Design review of the part built by this model. Coordinates are the model's own, in mm. Face numbers are marked on the shaded views. Round coordinates to 2 decimals unless told otherwise and drop trailing zeros. Write each loop counter-clockwise with the first axis right and the second up, starting at its lowest first coordinate (ties: lowest second). Pieces come first, ordered by that corner, then holes. Notation, with made-up numbers: M 25,-11.75 L 67,-11.75 A36 ccw 67,23.25 Z; hole C 85,-34 d8. An arc over 180 degrees is marked long. One line per question, with ' | ' between items. Start each with the question number.
Item 1: Add section B-B, the plane z = 0. State the section outline as (x, y) points, and give its area (3 significant figures).
Item 2: Add section C-C, the plane y = 16.5. State the section outline as (x, z) points.
Item 3: For L1, parallel to X at y = 5, z = 9; L2, parallel to Z at x = 10, y = 3; L3, parallel to Z at x = -9.5, y = 6, list the stretches that pass through material, from the lowest coordinate up.
Item 4: Draft analysis for pull direction X (two halves, no side actions). For the marked faces 1, 2 and 3, state which applies: released by +X, released by -X, zero draft, split by the parting line, or undercut.
Item 5: Insertion check: pin 1 Ø2 at (y, z) = (17, 16) entering from +X; pin 2 Ø6 at (y, z) = (10.5, -12.5) entering from -X; pin 3 Ø4 at (x, z) = (8.5, -12.5) entering from +Y. Each pin has a flat end and moves straight along its axis. Give the tip position at first contact, or say it passes through.
Item 6: Add section A-A, the plane y = 23.5. State the section outline as (x, z) points, and give its area (3 significant figures).
```python
from build123d import *

# Parameters (mm, degrees)
SKETCH2_R           = 22
BOSS_EXTRUDE3_DEPTH = 30
SKETCH1_R           = 4.5
CUT_EXTRUDE2_DEPTH  = 25
FILLET1_R           = 7.5
BOSS_EXTRUDE4_DEPTH = 1


with BuildPart() as part:
    # Sketch2 → Boss-Extrude3 (new body)
    with BuildSketch(Plane(origin=(0, 30, 0), x_dir=(1, 0, 0), z_dir=(0, 1, 0))):
        with Locations(Location((0, 0, 0), (0, 0, 270))):
            Circle(SKETCH2_R)
    extrude(amount=-BOSS_EXTRUDE3_DEPTH)

    # Sketch1 → Cut-Extrude2 (cut)
    with BuildSketch(Plane(origin=(0, 0, 0), x_dir=(1, 0, 0), z_dir=(0, 1, 0))):
        with Locations(Location((0, 13, 0), (0, 0, 270))):
            Circle(SKETCH1_R)
        with Locations(Location((-11.258330249, 6.5, 0), (0, 0, 270))):
            Circle(SKETCH1_R)
        with Locations(Location((-11.258330249, -6.5, 0), (0, 0, 270))):
            Circle(SKETCH1_R)
        with Locations(Location((11.258330249, 6.5, 0), (0, 0, 270))):
            Circle(SKETCH1_R)
        with Locations(Location((11.258330249, -6.5, 0), (0, 0, 270))):
            Circle(SKETCH1_R)
        with Locations(Location((0, -13, 0), (0, 0, 270))):
            Circle(SKETCH1_R)
    extrude(amount=CUT_EXTRUDE2_DEPTH, mode=Mode.SUBTRACT)

    # Fillet1
    fillet1_edges = [part.edges().sort_by_distance(p)[0] for p in [
        (0, 30, -22),
    ]]
    fillet(fillet1_edges, radius=FILLET1_R)

    # Sketch3 → Boss-Extrude4 (add)
    with BuildSketch(Plane(origin=(0, 30, 0), x_dir=(1, 0, 0), z_dir=(0, 1, 0))):
        with BuildLine():
            Line((-5.047435897, 6.7), (-3.907692308, 6.7))
            Line((-3.907692308, 6.7), (-3.907692308, -1.876061699))
            add(Edge.make_bspline(
                [(-3.907692308, -1.876061699), (-3.908831384, -2.034649033), (-3.911018549, -2.339156067), (-3.923045124, -2.777755632), (-3.945300887, -3.17824355), (-3.977722218, -3.541530486), (-4.020975634, -3.86647833), (-4.070473079, -4.155597886), (-4.130390949, -4.406476162), (-4.220620698, -4.688181596), (-4.368571883, -4.997131973), (-4.591246564, -5.330797805), (-4.867862712, -5.622656181), (-5.188269318, -5.876121783), (-5.555266748, -6.078078021), (-5.961297429, -6.22305824), (-6.403861903, -6.311489634), (-6.710836188, -6.320829233), (-6.868990385, -6.325641026)],
                knots=[0, 0, 0, 0, 1.237770943, 2.376671248, 3.424123796, 4.367912054, 5.222547132, 5.982086412, 6.656319012, 7.234008312, 8.288027371, 9.317870876, 10.352700517, 11.413286737, 12.494591526, 13.606319346, 14.766767577, 16, 16, 16, 16], degree=3))
            add(Edge.make_bspline(
                [(-6.868990385, -6.325641026), (-6.992210713, -6.321719958), (-7.240138175, -6.313830511), (-7.609130176, -6.249526009), (-7.977074488, -6.150407795), (-8.345924031, -6.00525552), (-8.722966135, -5.80784092), (-9.113307336, -5.549541728), (-9.521968629, -5.230838761), (-9.791147982, -4.987587513), (-9.932051282, -4.86025641)],
                knots=[0, 0, 0, 0, 0.848567217, 1.707373443, 2.573483905, 3.470863513, 4.432650262, 5.500696352, 6.691726801, 8, 8, 8, 8], degree=3))
            Line((-9.932051282, -4.86025641), (-9.260416667, -3.883333333))
            add(Edge.make_bspline(
                [(-9.260416667, -3.883333333), (-9.105466946, -3.990185314), (-8.812901668, -4.191935786), (-8.38289984, -4.451475164), (-8.00191017, -4.673997908), (-7.75268919, -4.787399035), (-7.637299679, -4.839903846)],
                knots=[0, 0, 0, 0, 1.196737151, 2.259595785, 3.194191475, 4, 4, 4, 4], degree=3))
            add(Edge.make_bspline(
                [(-7.637299679, -4.839903846), (-7.567325178, -4.867333877), (-7.430089597, -4.921130276), (-7.220267165, -4.98116825), (-7.011642317, -5.01397928), (-6.873329542, -5.020080117), (-6.805388622, -5.023076923)],
                knots=[0, 0, 0, 0, 1.051806502, 2.062826769, 3.048436908, 4, 4, 4, 4], degree=3))
            add(Edge.make_bspline(
                [(-6.805388622, -5.023076923), (-6.717639647, -5.019365856), (-6.544192277, -5.012030446), (-6.292137213, -4.947263075), (-6.050989499, -4.848404813), (-5.829393884, -4.703656404), (-5.625158337, -4.531548106), (-5.456637227, -4.323427732), (-5.31614894, -4.092774019), (-5.231604338, -3.8744376), (-5.177739023, -3.675313828), (-5.143551977, -3.492313592), (-5.113657409, -3.278367655), (-5.087598635, -3.033220643), (-5.072342413, -2.756381753), (-5.055225452, -2.448663863), (-5.049037791, -2.109291153), (-5.047986155, -1.872668556), (-5.047435897, -1.748858173)],
                knots=[0, 0, 0, 0, 0.997221856, 1.971139923, 2.944579524, 3.951425367, 4.971190333, 5.972282193, 6.985401279, 8.033996657, 8.624075553, 9.332086008, 10.151144245, 11.082816738, 12.137127781, 13.306538797, 14.590673636, 16, 16, 16, 16], degree=3))
            Line((-5.047435897, -1.748858173), (-5.047435897, 6.7))
        make_face()
        Polygon((-0.651282051, -6), (-0.651282051, 6.7), (-0.412139423, 6.7), (7.978205128, -3.295653045), (7.978205128, 6.7), (9.117948718, 6.7), (9.117948718, -6), (8.858453526, -6), (0.488461538, 3.97275641), (0.488461538, -6), align=None)
    extrude(amount=BOSS_EXTRUDE4_DEPTH)


solid = part.part
```
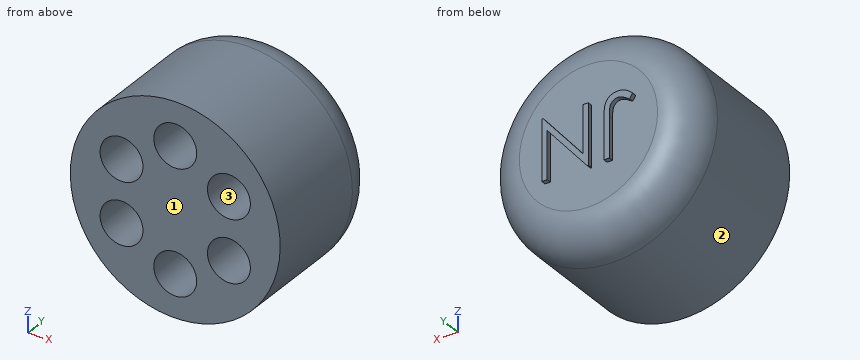
Computed values:
1) outline: M -22,0 L 22,0 L 22,22.5 A7.5 ccw 14.5,30 L 9.12,30 L 9.12,31 L 7.98,31 L 7.98,30 L 5.21,30 L 5.21,31 L 3.82,31 L 3.82,30 L 0.49,30 L 0.49,31 L -0.65,31 L -0.65,30 L -3.91,30 L -3.91,31 L -5.05,31 L -5.05,30 L -14.5,30 A7.5 ccw -22,22.5 Z | area: 1,300 mm^2
2) outline: C 0,0 d44; hole C -11.26,-6.5 d9; hole C -11.26,6.5 d9; hole C 0,-13 d9; hole C 0,13 d9; hole C 11.26,-6.5 d9; hole C 11.26,6.5 d9
3) L1: x = -20.07 to -15, -7.52 to -2.06, 2.06 to 7.52, 15 to 20.07 | L2: z = -19.6 to -10.82, -2.18 to 2.18, 10.82 to 19.6 | L3: z = -19.84 to -10.64, -2.36 to 2.36, 10.64 to 19.84
4) face 1: zero draft | face 2: split by the parting line | face 3: undercut
5) pin 1: stops at x = 16.09 | pin 2: stops at x = -19.84 | pin 3: stops at y = 30
6) outline: C 0,0 d43.87; hole C -11.26,-6.5 d9; hole C -11.26,6.5 d9; hole C 0,-13 d9; hole C 0,13 d9; hole C 11.26,-6.5 d9; hole C 11.26,6.5 d9 | area: 1,130 mm^2
